Geometry check sheet. Reference: the model listing, model coordinates, mm. A direction names the side the tool comes from. Coordinates: 2 decimals unless noted, no trailing zeros. Loops run counter-clockwise (first coordinate to the right, second up) from the corner with the lowest first, then second, coordinate; pieces in that order, holes last.
from build123d import *

# Parameters (mm, degrees)
SKETCH1_W               = 100
SKETCH1_H               = 40
SKETCH1_R               = 2.75
BOSS_EXTRUDE1_DEPTH     = 8
SKETCH2_R               = 5
BOSS_EXTRUDE2_DEPTH     = 40
BOSS_EXTRUDE3_START     = 4
SKETCH4_W               = 9.8
SKETCH4_H               = 40
SKETCH4_R               = 2.75
BOSS_EXTRUDE3_DEPTH     = 4
SKETCH5_R               = 5.25
CUT_EXTRUDE1_DEPTH      = 4
CHAMFER2_SIZE           = 2.5
CUT_EXTRUDE2_REACH      = 96.977
CUT_EXTRUDE2_END_RADIUS = 5
SKETCH6_R               = 1.4
BOSS_EXTRUDE4_DEPTH     = 40


# Some blends are built 0.0001 mm under size
with BuildPart() as part:
    # Sketch1 → Boss-Extrude1 (new body)
    with BuildSketch(Plane.XY):
        Rectangle(SKETCH1_W, SKETCH1_H)
        with Locations((-25, 0)):
            Circle(SKETCH1_R, mode=Mode.SUBTRACT)
        with Locations((25, 0)):
            Circle(SKETCH1_R, mode=Mode.SUBTRACT)
    extrude(amount=BOSS_EXTRUDE1_DEPTH)

    # Sketch2 → Boss-Extrude2 (add)
    with BuildSketch(Plane.XZ.offset(20)):
        with BuildLine():
            Line((-50, 0), (-59.9, 0))
            Line((-59.9, 0), (-59.9, 27.5))
            ThreePointArc((-59.9, 27.5), (-72.9, 40.5), (-59.9, 53.5))
            Line((-59.9, 53.5), (-51.9, 53.5))
            Line((-51.9, 53.5), (-51.9, 8))
            Line((-51.9, 8), (-50, 8))
            Line((-50, 8), (-50, 0))
        make_face()
        with Locations(Location((-59.9, 40.5, 0), (0, 0, 270))):
            Circle(SKETCH2_R, mode=Mode.SUBTRACT)
    extrude(amount=-BOSS_EXTRUDE2_DEPTH)

    # Chamfer1
    # the kernel refuses this chamfer: 10 mm, written as the material it adds along each edge
    with BuildSketch(Plane(origin=(-51.9, -20, 8), x_dir=(0.9996219169112968, 0, -0.027495876610586403), z_dir=(0, 1, 0))) as chamfer1_piece_1:
        with BuildLine():
            Line((10.286731952, 0), (-0.565471549, -10.271177935))
            Line((-0.565471549, -10.271177935), (-0.765395932, -10.26567876))
            ThreePointArc((-0.765395932, -10.26567876), (-0.341292271, -5.133978296), (-0.199924383, 0.005499175))
            Line((-0.199924383, 0.005499175), (0.005499175, 0.199924383))
            ThreePointArc((0.005499175, 0.199924383), (5.144976647, 0.058556496), (10.292231127, 0.199924383))
            Line((10.292231127, 0.199924383), (10.286731952, 0))
        make_face()
    extrude(amount=40)
    with BuildSketch(Plane(origin=(-59.9, -20, 27.5), x_dir=(-0.9634026382887829, 0, 0.26805849462050707), z_dir=(0, 1, 0))) as chamfer1_piece_2:
        with BuildLine():
            Line((6.087608123, 0), (-2.363030305, -7.699460597))
            Line((-2.363030305, -7.699460597), (-2.555710833, -7.645848898))
            ThreePointArc((-2.555710833, -7.645848898), (-1.271764875, -3.82461909), (-0.192680528, 0.053611699))
            Line((-0.192680528, 0.053611699), (0.053611699, 0.192680528))
            ThreePointArc((0.053611699, 0.192680528), (3.034373901, -0.267839497), (6.052113215, 0.196825079))
            Line((6.052113215, 0.196825079), (6.087608123, 0))
        make_face()
    extrude(amount=40)
    # the kernel refuses this chamfer: 10 mm, written as the material it takes off along each edge
    with BuildSketch(Plane(origin=(-59.9, -45.71682988, 0), x_dir=(-0.027495876610586324, 0, 0.9996219169112968), z_dir=(0, 1, 0))) as chamfer1_2_piece_1:
        with BuildLine():
            Line((10.286731952, 0), (-0.565471549, 10.271177935))
            Line((-0.565471549, 10.271177935), (-0.765395932, 10.26567876))
            ThreePointArc((-0.765395932, 10.26567876), (-0.341292271, 5.133978296), (-0.199924383, -0.005499175))
            Line((-0.199924383, -0.005499175), (0.005499175, -0.199924383))
            ThreePointArc((0.005499175, -0.199924383), (5.144976647, -0.058556496), (10.292231127, -0.199924383))
            Line((10.292231127, -0.199924383), (10.286731952, 0))
        make_face()
    extrude(amount=91.433659759, mode=Mode.SUBTRACT)

    # Sketch4 → Boss-Extrude3 (add)
    # profile 1 of 2: a face of its own
    with BuildSketch(Plane(origin=(0, 0, 0), x_dir=(-1, 0, 0), z_dir=(0, 0, -1)).offset(BOSS_EXTRUDE3_START)):
        with Locations((25, 0)):
            Rectangle(SKETCH4_W, SKETCH4_H)
        with Locations((25, 0)):
            Circle(SKETCH4_R, mode=Mode.SUBTRACT)
    # profile 2 of 2: a face of its own
    with BuildSketch(Plane(origin=(0, 0, 0), x_dir=(-1, 0, 0), z_dir=(0, 0, -1)).offset(BOSS_EXTRUDE3_START)):
        with Locations((-25, 0)):
            Rectangle(SKETCH4_W, SKETCH4_H)
        with Locations(Location((-25, 0, 0), (0, 0, 180))):
            Circle(SKETCH4_R, mode=Mode.SUBTRACT)
    extrude(amount=-BOSS_EXTRUDE3_DEPTH)

    # Sketch5 → Cut-Extrude1 (cut)
    with BuildSketch(Plane.XY.offset(8)):
        with Locations((25, 0)):
            Circle(SKETCH5_R)
        with Locations((-25, 0)):
            Circle(SKETCH5_R)
    extrude(amount=-CUT_EXTRUDE1_DEPTH, mode=Mode.SUBTRACT)

    # Chamfer2
    chamfer2_edges = [part.edges().sort_by_distance(p)[0] for p in [
        (22.25, 0, 4),
        (-27.75, 0, 4),
    ]]
    chamfer(chamfer2_edges, length=CHAMFER2_SIZE - 0.0001)  # a hair under: the kernel refuses the full size

    # Cut-Extrude2: up to this cylinder (the profile starts outside it)
    cut_extrude2_end = Plane(origin=(-59.9, 0, 40.5), z_dir=(0, -1, 0)) * Cylinder(CUT_EXTRUDE2_END_RADIUS, 204.954, mode=Mode.PRIVATE)
    # Sketch6 → Cut-Extrude2 (cut, up to the surface)
    with BuildSketch(Plane.XY.offset(53.5), mode=Mode.PRIVATE) as cut_extrude2_sk1:
        with Locations((-59.9, 0)):
            Circle(SKETCH6_R)
    cut_extrude2_tool1 = extrude(cut_extrude2_sk1.sketch, amount=-CUT_EXTRUDE2_REACH, mode=Mode.PRIVATE) - cut_extrude2_end
    add(cut_extrude2_tool1.solids().sort_by_distance((-59.9, 0, 53.5))[0], mode=Mode.SUBTRACT)

    # Sketch7 → Boss-Extrude4 (add)
    with BuildSketch(Plane.XZ.offset(20)):
        Polygon((-59.9, 10), (-71.659995777, 34.959016393), (-59.9, 34.959016393), align=None)
    extrude(amount=-BOSS_EXTRUDE4_DEPTH)


solid = part.part
1) Section check B-B on y = 8.5. Record the cut outline in (x, z).
Data:
outline: (-71.66, 34.96) - (-59.9, 10) - (-49.9, 0) - (-29.9, 0) - (-29.9, -4) - (-20.1, -4) - (-20.1, 0) - (20.1, 0) - (20.1, -4) - (29.9, -4) - (29.9, 0) - (50, 0) - (50, 8) - (-41.9, 8) - (-51.9, 18) - (-51.9, 53.5) - (-59.9, 53.5) arc R13 ccw to start; hole circle Ø10 at (-59.9, 40.5)
2) Depth check by flat-ended pin: pin 1 (18 mm diameter, centred on y = 2.5, z = 32, fed in from +X); pin 2 (9 mm diameter, centred on x = 25, y = 0, fed in from +Z); pin 3 (8 mm diameter, centred on x = -32.5, y = -6.5, fed in from +Z); pin 4 (3 mm diameter, centred on x = -48.5, z = 26, fed in from +Y). Enter the tip coordinate at first touch or a pass-through.
Data:
pin 1: stops at x = -51.9
pin 2: stops at z = 3.25
pin 3: stops at z = 8
pin 4: passes through
3) Mould release check, pull along X, two halves, no side actions. Record for faces 6 (the flat face through (-20.1, 0, -2)), 7 (the flat face through (-51.9, 0, 36)), 8 (the cylindrical face through (-70.975, -0.28, 47.308)): +X half, -X half, draft (parallel to the pull), parting line (faces both ways), or undercut.
Data:
face 6: undercut
face 7: +X half
face 8: -X half
4) Section check A-A on z = 40.5. Record the cut outline in (x, y).
Data:
outline: (-72.9, -20) - (-64.9, -20) - (-64.9, 20) - (-72.9, 20) - close; (-54.9, -20) - (-51.9, -20) - (-51.9, 20) - (-54.9, 20) - close
5) Section check D-D on x = -45. Record the cut outline in (y, z).
Data:
outline: (-20, 0) - (20, 0) - (20, 11.1) - (-20, 11.1) - close
6) Material ranges on probe 1 along X at (y, z) = (0, 0.85); probe 2 along Y at (x, z) = (-25, 5.3); probe 3 along Z at (x, y) = (20, -12), recorded low to high.
Data:
probe 1: x = -50.75 to -27.75, -22.25 to 22.25, 27.75 to 50
probe 2: y = -20 to -5.25, 5.25 to 20
probe 3: z = 0 to 8
7) Access from +Z, -Z, +X, -X, +Y, -Y to the whole of each face (thin tool, end or side, straight path). Record for faces 1 (the flat face through (3, 0, 8)), 2 (the cylindrical face through (19.755, 0.231, 6.028)), 3 (the flat face through (-56, 0, 53.5)), 4 (the flat face through (-40, 0, 0)), 5 (the flat face through (20.1, 0, -2)).
Data:
face 1: +Z, +X, +Y, -Y
face 2: +Z
face 3: +Z, +X, -X, +Y, -Y
face 4: -Z, -X, +Y, -Y
face 5: -Z, +Y, -Y
